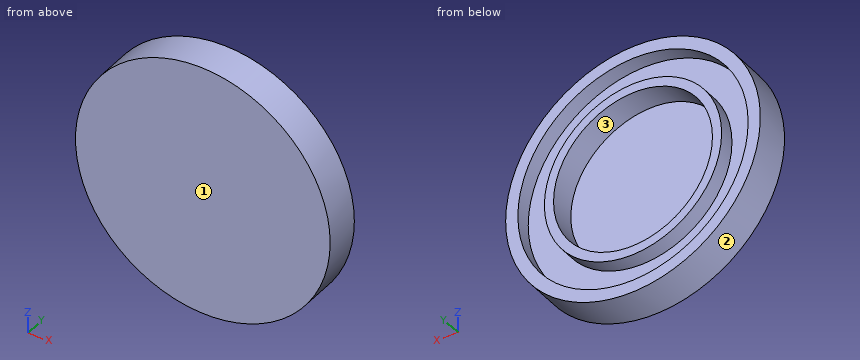
```python
from build123d import *

# Parameters (mm, degrees)
ESQUISSE2_R             = 25
BOSS_EXTRU_1_DEPTH      = 7
ESQUISSE3_R             = 15.6
ENL_V_MAT_EXTRU_1_DEPTH = 5
ESQUISSE5_R             = 22.6
ESQUISSE5_R_2           = 17.4
ENL_V_MAT_EXTRU_2_DEPTH = 3


with BuildPart() as part:
    # Esquisse2 → Boss.-Extru.1 (new body)
    with BuildSketch(Plane(origin=(0, 0, 0), x_dir=(1, 0, 0), z_dir=(0, 1, 0))):
        Circle(ESQUISSE2_R)
    extrude(amount=BOSS_EXTRU_1_DEPTH)

    # Esquisse3 → Enlèv. mat.-Extru.1 (cut)
    with BuildSketch(Plane(origin=(0, 7, 0), x_dir=(1, 0, 0), z_dir=(0, 1, 0))):
        Circle(ESQUISSE3_R)
    extrude(amount=-ENL_V_MAT_EXTRU_1_DEPTH, mode=Mode.SUBTRACT)

    # Esquisse5 → Enlèv. mat.-Extru.2 (cut)
    with BuildSketch(Plane(origin=(0, 7, 0), x_dir=(1, 0, 0), z_dir=(0, 1, 0))):
        Circle(ESQUISSE5_R)
        Circle(ESQUISSE5_R_2, mode=Mode.SUBTRACT)
    extrude(amount=-ENL_V_MAT_EXTRU_2_DEPTH, mode=Mode.SUBTRACT)


solid = part.part
```
Geometry: final body of the model. Coordinates: model frame, mm. Face numbers are marked on the shaded views. Round coordinates to 2 decimals unless told otherwise and drop trailing zeros. Order: outer loops, then holes, each group sorted by start corner. A loop starts at its lowest first (then second) coordinate and runs counter-clockwise, first axis right, second up. Notation, with made-up numbers: (22, 69) -> (43, 69) arc R6 cw to (43, 79) -> close; hole circle Ø9 at (31.5, -9). An arc over 180 degrees is marked (long way). Write each question's results on one line, items separated by ' | '.
Q1. Section query A-A (y = 5.25). Output: boundary loops of the cut face in (x, z).
Response values:
outline: circle Ø50 at (0, 0); circle Ø34.8 at (0, 0); hole circle Ø45.2 at (0, 0); hole circle Ø31.2 at (0, 0)
Q2. Ray query, line 1 along Z through (x, y) = (0, 5.2); line 2 along Z through (x, y) = (0, 3.3); line 3 along X through (y, z) = (6.75, 6). Return the intervals inside material, ascending.
Response values:
line 1: -25 to -22.6, -17.4 to -15.6, 15.6 to 17.4, 22.6 to 25 | line 2: -25 to -15.6, 15.6 to 25 | line 3: -24.27 to -21.79, -16.33 to -14.4, 14.4 to 16.33, 21.79 to 24.27
Q3. Section query B-B (z = 0). Output: boundary loops of the cut face in (x, y), and give its area (3 significant figures).
Response values:
outline: (-25, 0) -> (25, 0) -> (25, 7) -> (22.6, 7) -> (22.6, 4) -> (17.4, 4) -> (17.4, 7) -> (15.6, 7) -> (15.6, 2) -> (-15.6, 2) -> (-15.6, 7) -> (-17.4, 7) -> (-17.4, 4) -> (-22.6, 4) -> (-22.6, 7) -> (-25, 7) -> close | area: 163 mm²
Q4. Pull-direction query (Z, two-part tool) for the marked faces 1, 2 and 3; classes: released by +Z, released by -Z, zero draft, split by the parting line, or undercut.
Response values:
face 1: zero draft | face 2: split by the parting line | face 3: undercut
Q5. Section query C-C (x = 0). Output: boundary loops of the cut face in (y, z), and give its area (3 significant figures).
Response values:
outline: (0, -25) -> (7, -25) -> (7, -22.6) -> (4, -22.6) -> (4, -17.4) -> (7, -17.4) -> (7, -15.6) -> (2, -15.6) -> (2, 15.6) -> (7, 15.6) -> (7, 17.4) -> (4, 17.4) -> (4, 22.6) -> (7, 22.6) -> (7, 25) -> (0, 25) -> close | area: 163 mm²
Q6. Pin query (flat end, axial travel): pin 1 Ø2 at (x, y) = (-4, 5.5) entering from +Z; pin 2 Ø2 at (y, z) = (4, 8.5) entering from +X; pin 3 Ø1 at (y, z) = (5.5, -6.5) entering from -X. Return the tip coordinate at first contact, or that it passes through.
Response values:
pin 1: z = 24.82 | pin 2: x = 23.85 | pin 3: x = -24.27
